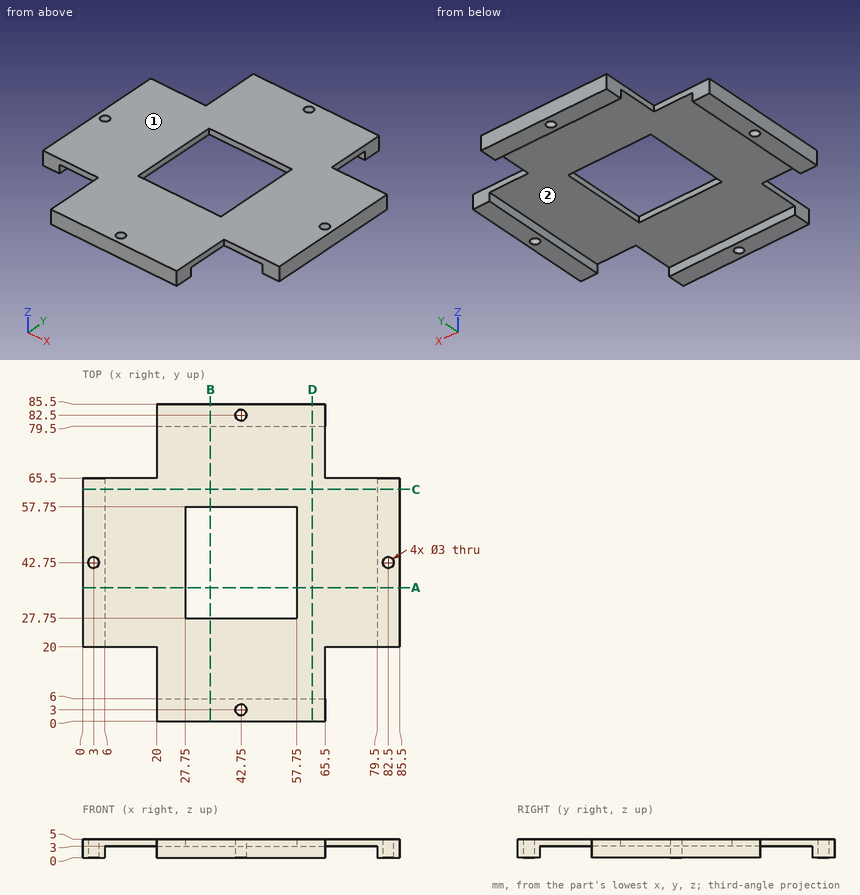
Part print with two shaded views. Sizes in mm from the minimum x, y, z corner. Round coordinates to 2 decimals unless told otherwise and drop trailing zeros. Order: outer loops, then holes, each group sorted by start corner. A loop starts at its lowest first (then second) coordinate and runs counter-clockwise, first axis right, second up. Notation, with made-up numbers: M -37,-38 L -19,-38 A30 cw -19,-10 Z; hole C 77.5,72.5 d4. An arc over 180 degrees is marked long. Use CSV: the item, a comma, the result in double quotes.
Item 1: Pull direction X, two halves, no side cores. Call the marked faces 1 and 2: released by +X, released by -X, zero draft, split by the parting line, or undercut.
Worked answers:
face 1,"zero draft"
face 2,"undercut"
Item 2: Pin check, flat tips, straight feed: pin 1 (1.6 mm diameter, centred on x = 43, z = 3.5, fed in from -Y); pin 2 (1.5 mm diameter, centred on y = 79.5, z = 3.5, fed in from -X); pin 3 (2.5 mm diameter, centred on x = 7, z = 2.5, fed in from -Y); pin 4 (6 mm diameter, centred on x = 74, y = 39.5, fed in from -Z). Stop position of each tip, or through.
Worked answers:
pin 1,"y = 0"
pin 2,"x = 20"
pin 3,"y = 20"
pin 4,"z = 3"
Item 3: Probe probe 1 along Y at (x, z) = (42.75, 2.1); probe 2 along X at (y, z) = (42.75, 3.15). List the from-to ranges inside material, lowest first.
Worked answers:
probe 1,"0 to 1.5, 4.5 to 6, 79.5 to 81, 84 to 85.5"
probe 2,"0 to 1.5, 4.5 to 27.75, 57.75 to 81, 84 to 85.5"
Item 4: Saw through at C-C (y = 62.5). List the corners of the cut face in (x, z), plus the area to 3 significant figures.
Worked answers:
outline,"M 0,0 L 6,0 L 6,3 L 79.5,3 L 79.5,0 L 85.5,0 L 85.5,5 L 0,5 Z"
area,"207 mm²"
Item 5: Saw through at A-A (y = 36). List the corners of the cut face in (x, z), plus the area to 3 significant figures.
Worked answers:
outline,"M 0,0 L 6,0 L 6,3 L 27.75,3 L 27.75,5 L 0,5 Z; M 57.75,3 L 79.5,3 L 79.5,0 L 85.5,0 L 85.5,5 L 57.75,5 Z"
area,"147 mm²"
